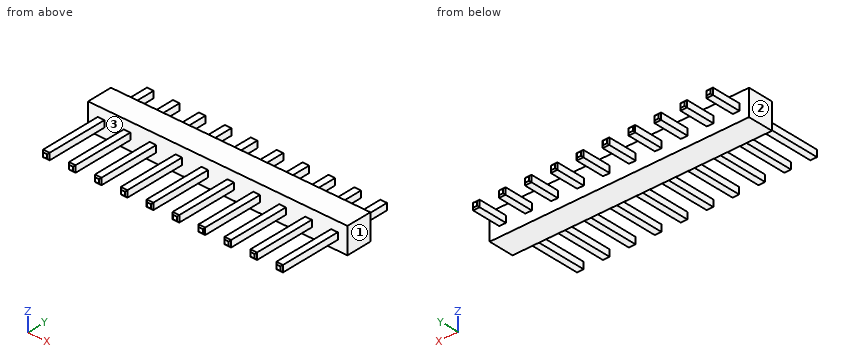
```python
from build123d import *

# Parameters (mm, degrees)
SKETCH3_W           = 25.4
SKETCH3_H           = 2.54
BOSS_EXTRUDE1_DEPTH = 2.5
SKETCH4_W           = 0.65
SKETCH4_H           = 0.65
BOSS_EXTRUDE2_DEPTH = 3
SKETCH5_W           = 0.65
SKETCH5_H           = 0.65
BOSS_EXTRUDE3_DEPTH = 6.1
CHAMFER1_SIZE       = 0.125


with BuildPart() as part:
    # Sketch3 → Boss-Extrude1 (new body)
    with BuildSketch(Plane(origin=(0, 0, 0), x_dir=(1, 0, 0), z_dir=(0, 1, 0))):
        Rectangle(SKETCH3_W, SKETCH3_H)
    extrude(amount=BOSS_EXTRUDE1_DEPTH)

    # Sketch4 → Boss-Extrude2 (add)
    with BuildSketch(Plane(origin=(0, 2.5, 0), x_dir=(1, 0, 0), z_dir=(0, 1, 0))):
        with Locations((1.27, 0)):
            Rectangle(SKETCH4_W, SKETCH4_H)
        with Locations((3.81, 0)):
            Rectangle(SKETCH4_W, SKETCH4_H)
        with Locations((6.35, 0)):
            Rectangle(SKETCH4_W, SKETCH4_H)
        with Locations((8.89, 0)):
            Rectangle(SKETCH4_W, SKETCH4_H)
        with Locations((11.43, 0)):
            Rectangle(SKETCH4_W, SKETCH4_H)
        with Locations((-3.81, 0)):
            Rectangle(SKETCH4_W, SKETCH4_H)
        with Locations((-6.35, 0)):
            Rectangle(SKETCH4_W, SKETCH4_H)
        with Locations((-1.27, 0)):
            Rectangle(SKETCH4_W, SKETCH4_H)
        with Locations((-8.89, 0)):
            Rectangle(SKETCH4_W, SKETCH4_H)
        with Locations((-11.43, 0)):
            Rectangle(SKETCH4_W, SKETCH4_H)
    extrude(amount=BOSS_EXTRUDE2_DEPTH)

    # Sketch5 → Boss-Extrude3 (add)
    with BuildSketch(Plane.XZ):
        with Locations((1.27, 0)):
            Rectangle(SKETCH5_W, SKETCH5_H)
        with Locations((3.81, 0)):
            Rectangle(SKETCH5_W, SKETCH5_H)
        with Locations((6.35, 0)):
            Rectangle(SKETCH5_W, SKETCH5_H)
        with Locations((8.89, 0)):
            Rectangle(SKETCH5_W, SKETCH5_H)
        with Locations((11.43, 0)):
            Rectangle(SKETCH5_W, SKETCH5_H)
        with Locations((-3.81, 0)):
            Rectangle(SKETCH5_W, SKETCH5_H)
        with Locations((-6.35, 0)):
            Rectangle(SKETCH5_W, SKETCH5_H)
        with Locations((-1.27, 0)):
            Rectangle(SKETCH5_W, SKETCH5_H)
        with Locations((-8.89, 0)):
            Rectangle(SKETCH5_W, SKETCH5_H)
        with Locations((-11.43, 0)):
            Rectangle(SKETCH5_W, SKETCH5_H)
    extrude(amount=BOSS_EXTRUDE3_DEPTH)

    # Chamfer1
    chamfer1_edges = [part.edges().sort_by_distance(p)[0] for p in [
        (-8.565, 5.5, 0),
        (-8.89, 5.5, -0.325),
        (-9.215, 5.5, 0),
        (-8.89, 5.5, 0.325),
        (-11.105, 5.5, 0),
        (-11.43, 5.5, -0.325),
        (-11.755, 5.5, 0),
        (-11.43, 5.5, 0.325),
        (1.595, -6.1, 0),
        (1.27, -6.1, 0.325),
        (0.945, -6.1, 0),
        (1.27, -6.1, -0.325),
        (4.135, -6.1, 0),
        (3.81, -6.1, 0.325),
        (3.485, -6.1, 0),
        (3.81, -6.1, -0.325),
        (6.675, -6.1, 0),
        (6.35, -6.1, 0.325),
        (6.025, -6.1, 0),
        (6.35, -6.1, -0.325),
        (9.215, -6.1, 0),
        (8.89, -6.1, 0.325),
        (8.565, -6.1, 0),
        (8.89, -6.1, -0.325),
        (1.595, 5.5, 0),
        (1.27, 5.5, -0.325),
        (0.945, 5.5, 0),
        (11.755, -6.1, 0),
        (11.43, -6.1, 0.325),
        (11.105, -6.1, 0),
        (11.43, -6.1, -0.325),
        (1.27, 5.5, 0.325),
        (-3.485, -6.1, 0),
        (-3.81, -6.1, 0.325),
        (-4.135, -6.1, 0),
        (-3.81, -6.1, -0.325),
        (-0.945, -6.1, 0),
        (-1.27, -6.1, 0.325),
        (-1.595, -6.1, 0),
        (-1.27, -6.1, -0.325),
        (-6.025, -6.1, 0),
        (-6.35, -6.1, 0.325),
        (-6.675, -6.1, 0),
        (-6.35, -6.1, -0.325),
        (-8.565, -6.1, 0),
        (-8.89, -6.1, 0.325),
        (-9.215, -6.1, 0),
        (-8.89, -6.1, -0.325),
        (-11.105, -6.1, 0),
        (-11.43, -6.1, 0.325),
        (-11.755, -6.1, 0),
        (-11.43, -6.1, -0.325),
        (-3.485, 5.5, 0),
        (-3.81, 5.5, -0.325),
        (-4.135, 5.5, 0),
        (-3.81, 5.5, 0.325),
        (4.135, 5.5, 0),
        (3.81, 5.5, -0.325),
        (3.485, 5.5, 0),
        (3.81, 5.5, 0.325),
        (6.675, 5.5, 0),
        (6.35, 5.5, -0.325),
        (6.025, 5.5, 0),
        (6.35, 5.5, 0.325),
        (9.215, 5.5, 0),
        (8.89, 5.5, -0.325),
        (8.565, 5.5, 0),
        (8.89, 5.5, 0.325),
        (11.755, 5.5, 0),
        (11.43, 5.5, -0.325),
        (11.105, 5.5, 0),
        (11.43, 5.5, 0.325),
        (-0.945, 5.5, 0),
        (-1.27, 5.5, -0.325),
        (-1.595, 5.5, 0),
        (-1.27, 5.5, 0.325),
        (-6.025, 5.5, 0),
        (-6.35, 5.5, -0.325),
        (-6.675, 5.5, 0),
        (-6.35, 5.5, 0.325),
    ]]
    chamfer(chamfer1_edges, length=CHAMFER1_SIZE)


solid = part.part
```
The model under review builds one solid part; all positions refer to its coordinate system, in mm. Face numbers are marked on the shaded views. Round coordinates to 2 decimals unless told otherwise and drop trailing zeros. Order: outer loops, then holes, each group sorted by start corner. A loop starts at its lowest first (then second) coordinate and runs counter-clockwise, first axis right, second up. Notation, with made-up numbers: (89, 43) -> (139, 43) arc R6 ccw to (139, 48) -> close; hole circle Ø2 at (13.5, -13.5). An arc over 180 degrees is marked (long way). Use a Markdown table: item, result.
Q1. Clearance check with flat-ended pins moving along their axes: P1, Ø0.5, axis at x = 11.5, y = -2.5, coming from the +Z side (3 decimals); P2, Ø0.7, axis at y = -1.5, z = 0, coming from the -X side (3 decimals); P3, Ø0.7, axis at y = 4.5, z = 0, coming from the +X side (3 decimals). State where each tip first meets the part, or that it passes through.
Values:
| item | result |
|---|---|
| P1 | stops at z = 0.325 |
| P2 | stops at x = -11.755 |
| P3 | stops at x = 11.755 |
Q2. We need section A-A on y = -4.5. State how many separate pieces and enclosed holes the cut face has, then the cut area to 4 significant figures.
Values:
| item | result |
|---|---|
| separate pieces | 10 |
| enclosed holes | 0 |
| area | 4.225 mm^2 |
Q3. We need section B-B on z = -0.85. Write out the cut boundary in (x, y), then the cut area to 3 significant figures.
Values:
| item | result |
|---|---|
| outline | (-12.7, 0) -> (12.7, 0) -> (12.7, 2.5) -> (-12.7, 2.5) -> close |
| area | 63.5 mm^2 |
Q4. Mouldability with a two-part tool opening along X and no side actions: class the marked faces 1, 2 and 3 as +X half, -X half, draft (parallel to the pull), parting line (faces both ways), or undercut.
Values:
| item | result |
|---|---|
| face 1 | +X half |
| face 2 | -X half |
| face 3 | undercut |
Q5. For line 1 (Y direction, x = 5, z = -0.4); line 2 (Z direction, x = -6.5, y = 3.25) (3 decimals); line 3 (Y direction, x = -11.5, z = 0.25), list the stretches that pass through material, from the lowest coordinate up.
Values:
| item | result |
|---|---|
| line 1 | y = 0 to 2.5 |
| line 2 | z = -0.325 to 0.325 |
| line 3 | y = -6.05 to 5.45 |
Q6. We need section C-C on x = -5.25. Write out the cut boundary in (y, z), then the cut area to 3 significant figures.
Values:
| item | result |
|---|---|
| outline | (0, -1.27) -> (2.5, -1.27) -> (2.5, 1.27) -> (0, 1.27) -> close |
| area | 6.35 mm^2 |
